Can you work these out from the model? Positions are in its coordinate system, mm. Face numbers are marked on the shaded views. A direction names the side the tool comes from. Round coordinates to 2 decimals unless told otherwise and drop trailing zeros. Order: outer loops, then holes, each group sorted by start corner. A loop starts at its lowest first (then second) coordinate and runs counter-clockwise, first axis right, second up. Notation, with made-up numbers: (17.25, -3.5) -> (54.25, -3.5) arc R16 ccw to (54.25, 25.5) -> close; hole circle Ø8 at (-27.5, 42.25). An arc over 180 degrees is marked (long way). One line per item, written item: value.
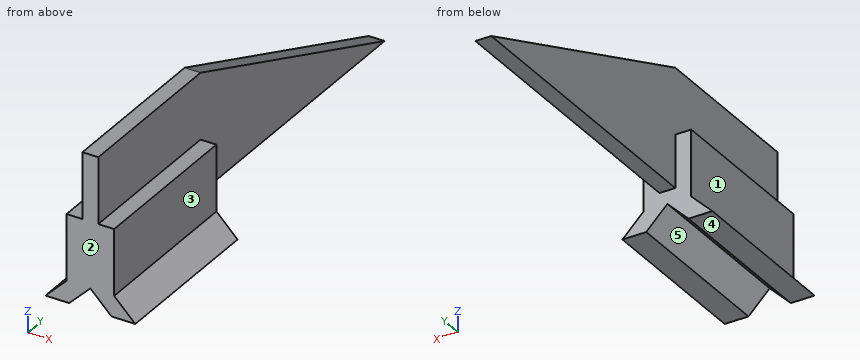
```python
from build123d import *

# Parameters (mm, degrees)
PAD_DEPTH         = 0.6
PAD001_DEPTH      = 12.5
SKETCH002_W       = 30
SKETCH002_H       = 1
POCKET_DEPTH      = 3.401
POCKET_DEPTH_BACK = 3.401


with BuildPart() as part:
    # Sketch → Pad (new body, symmetric)
    with BuildSketch(Plane.YZ):
        Polygon((0, 0), (-12.5, 0), (-12.5, 10), (0, 10), (25, 0), align=None)
    extrude(amount=PAD_DEPTH, both=True)

    # Sketch001 → Pad001 (join)
    with BuildSketch(Plane.XZ):
        Polygon((1.8, 0), (3.4, -1.6), (1.6, -1.6), (0, 0), (-1.6, -1.6), (-3.4, -1.6), (-1.8, 0), (-1.8, 5), (1.8, 5), align=None)
    extrude(amount=PAD001_DEPTH)

    # Sketch002 → Pocket (cut, two sides)
    with BuildSketch(Plane.YZ) as pocket_sk:
        with Locations((15, 0.5)):
            Rectangle(SKETCH002_W, SKETCH002_H)
    extrude(amount=-POCKET_DEPTH, mode=Mode.SUBTRACT)
    extrude(pocket_sk.sketch, amount=POCKET_DEPTH_BACK, mode=Mode.SUBTRACT)


solid = part.part
```
Q1. Please list where these lines run through material, in increasing order: line 1 along Y through (x, z) = (1, 2.5); line 2 along X through (y, z) = (13.5, 3.75); line 3 along X through (y, z) = (-3, 1.5).
Answers below:
line 1: -12.5 to 0
line 2: -0.6 to 0.6
line 3: -1.8 to 1.8
Q2. I want a section at B-B on y = -6. List the corners of the cut face in (x, z) for me, plus the area to 3 significant figures.
Answers below:
outline: (-3.4, -1.6) -> (-1.6, -1.6) -> (0, 0) -> (1.6, -1.6) -> (3.4, -1.6) -> (1.8, 0) -> (1.8, 5) -> (0.6, 5) -> (0.6, 10) -> (-0.6, 10) -> (-0.6, 5) -> (-1.8, 5) -> (-1.8, 0) -> close
area: 29.8 mm^2
Q3. We'd pull the mould along X, two halves only. Please class the marked faces 3, 4 and 5: released by +X, released by -X, zero draft, split by the parting line, or undercut.
Answers below:
face 3: released by +X
face 4: zero draft
face 5: undercut
Q4. I want a section at C-C on z = 2. List the corners of the cut face in (x, y) for me, plus the area to 3 significant figures.
Answers below:
outline: (-1.8, -12.5) -> (1.8, -12.5) -> (1.8, 0) -> (0.6, 0) -> (0.6, 20) -> (-0.6, 20) -> (-0.6, 0) -> (-1.8, 0) -> close
area: 69.0 mm^2
Q5. On a 3-axis mill with a long thin cutter (end or side, diameter ignored), from which of +Z, -Z, +X, -X, +Y, -Y can I reach the whole of each face in a straight line? I mean the marked faces 1 and 2. Say none if no direction works.
Answers below:
face 1: +Z, -X, +Y, -Y
face 2: +Z, -Z, +X, -X, -Y
Q6. I want a section at D-D on x = -1. List the corners of the cut face in (y, z) for me.
Answers below:
outline: (-12.5, -1) -> (0, -1) -> (0, 5) -> (-12.5, 5) -> close
Q7. Will these pins go through, and if not, where does the flat tip stop? pin 1 Ø1.3 at (x, y) = (1.5, -6.5) entering from +Z; pin 2 Ø2.5 at (y, z) = (4, 6) entering from -X; pin 3 Ø5 at (y, z) = (0, 3.5) entering from -X; pin 4 Ø1 at (x, y) = (-2, 7) entering from -Z.
Answers below:
pin 1: z = 5
pin 2: x = -0.6
pin 3: x = -1.8
pin 4: through
Q8. I want a section at A-A on z = -0.5. List the corners of the cut face in (x, y) for me, plus the area to 3 significant figures.
Answers below:
outline: (-2.3, -12.5) -> (-0.5, -12.5) -> (-0.5, 0) -> (-2.3, 0) -> close; (0.5, -12.5) -> (2.3, -12.5) -> (2.3, 0) -> (0.5, 0) -> close
area: 45.0 mm^2
